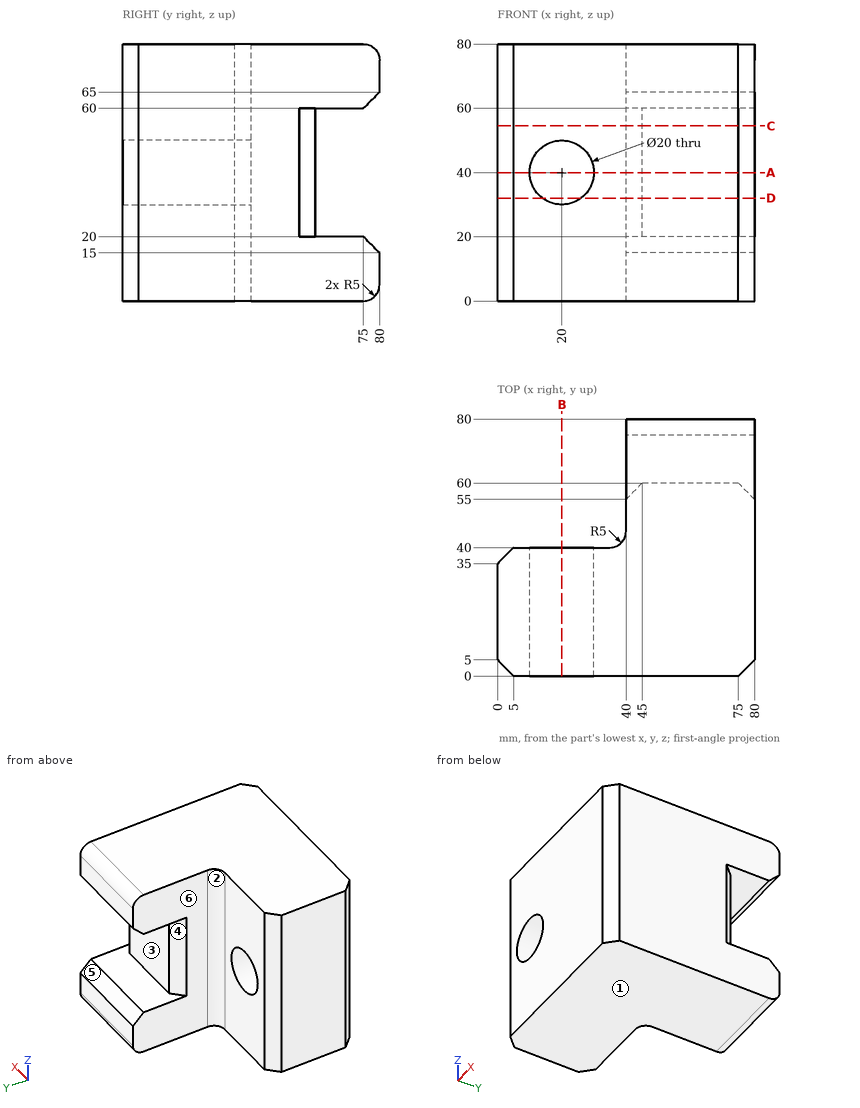
Could you check a few things on this drawing? It's one solid part, dimensions in mm from its lowest x, y, z. A direction names the side the tool comes from. Round coordinates to 2 decimals unless told otherwise and drop trailing zeros. Loops run counter-clockwise (first coordinate to the right, second up) from the corner with the lowest first, then second, coordinate; pieces in that order, holes last.
Q1. I want a section at A-A (z = 40). Write out the boundary of the cut face in (x, y), and give its area (3 significant figures).
Q2. On a 3-axis mill with a long thin cutter (end or side, diameter ignored), from which of +Z, -Z, +X, -X, +Y, -Y can I reach the whole of each face in a straight line? I mean the marked faces 4, 5 and 6. Say none if no direction works.
Q3. Please list where these lines run through material, in increasing order: L1, parallel to X at y = 22, z = 40; L2, parallel to Z at x = 54, y = 66; L3, parallel to Y at x = 25, z = 60.5.
Q4. I want a section at B-B (x = 20). Write out the boundary of the cut face in (y, z).
Q5. For P1, Ø1, axis at x = 68, z = 40.5, coming from the +Y side; P2, Ø15, axis at x = 24, z = 36, coming from the +Y side; P3, Ø2, axis at y = 46.5, z = 46, coming from the -X side; P4, Ø10, axis at y = 31.5, z = 30.5, coming from the -X side, each with a flat end and sliding along its axis, tell me the tip position at first contact or that it passes through.
Q6. Thinking about a two-plate mould opening in Z: for the marked faces 1, 2 and 3, which applies, pulls with the +Z half, pulls with the -Z half, needs draft (parallel to the pull), parting line crosses it, or undercut?
Q7. I want a section at C-C (z = 54.5). Write out the boundary of the cut face in (x, y).
Q8. I want a section at D-D (z = 32). Write out the boundary of the cut face in (x, y), and give its area (3 significant figures).
Answer below:
1. outline: (0, 5) - (5, 0) - (10, 0) - (10, 40) - (5, 40) - (0, 35) - close; (30, 0) - (75, 0) - (80, 5) - (80, 55) - (75, 60) - (45, 60) - (40, 55) - (40, 45) arc R5 cw to (35, 40) - (30, 40) - close
1. area: 3,140 mm2
2. face 4: -X, +Y
2. face 5: +X, -X, +Y
2. face 6: +Z, -Z, -X, +Y
3. L1: x = 0 to 10, 30 to 80
3. L2: z = 0 to 20, 60 to 80
3. L3: y = 0 to 40
4. outline: (0, 0) - (40, 0) - (40, 30) - (0, 30) - close; (0, 50) - (40, 50) - (40, 80) - (0, 80) - close
5. P1: stops at y = 60
5. P2: stops at y = 40
5. P3: stops at x = 40
5. P4: stops at x = 0
6. face 1: pulls with the -Z half
6. face 2: needs draft
6. face 3: undercut
7. outline: (0, 5) - (5, 0) - (75, 0) - (80, 5) - (80, 55) - (75, 60) - (45, 60) - (40, 55) - (40, 45) arc R5 cw to (35, 40) - (5, 40) - (0, 35) - close
8. outline: (0, 5) - (5, 0) - (14, 0) - (14, 40) - (5, 40) - (0, 35) - close; (26, 0) - (75, 0) - (80, 5) - (80, 55) - (75, 60) - (45, 60) - (40, 55) - (40, 45) arc R5 cw to (35, 40) - (26, 40) - close
8. area: 3,460 mm2
